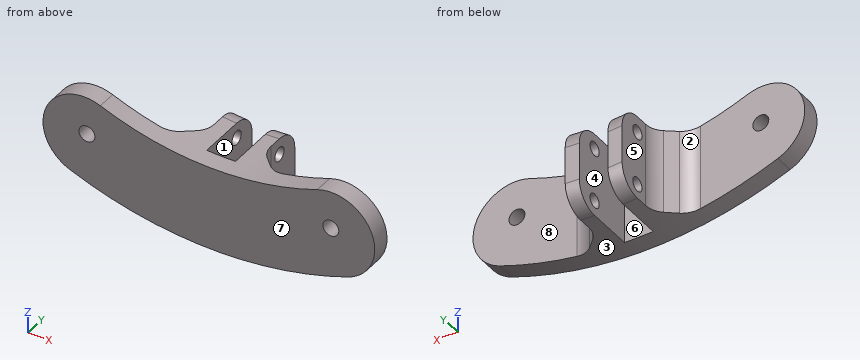
from build123d import *

# Parameters (mm, degrees)
SKETCH1_R               = 1.7
BOSS_EXTRUDE1_DEPTH     = 18.75
SKETCH2_W               = 29.270887873
SKETCH2_H               = 14.75
SKETCH2_W_2             = 6.11
CUT_EXTRUDE1_DEPTH      = 91.963568829
CHAMFER1_SIZE           = 5
FILLET1_R               = 5
CUT_EXTRUDE2_DEPTH      = 93.192977357
CUT_EXTRUDE2_DEPTH_BACK = 93.192977357
SKETCH4_R               = 1.5
FILLET2_R               = 5


with BuildPart() as part:
    # Sketch1 → Boss-Extrude1 (new body)
    with BuildSketch(Plane(origin=(0, 0, 0), x_dir=(1, 0, 0), z_dir=(0, 1, 0))):
        with BuildLine():
            ThreePointArc((-23.098921993, 59.418030115), (0, 63.75), (23.098921993, 59.418030115))
            ThreePointArc((23.098921993, 59.418030115), (34.716014466, 64.531190827), (29.602853754, 76.148283301))
            ThreePointArc((29.602853754, 76.148283301), (0, 81.7), (-29.602853754, 76.148283301))
            ThreePointArc((-29.602853754, 76.148283301), (-34.716014466, 64.531190827), (-23.098921993, 59.418030115))
        make_face()
        with Locations(Location((-25.965, 66.790526087, 0), (0, 0, 270))):
            Circle(SKETCH1_R, mode=Mode.SUBTRACT)
        with Locations(Location((25.965, 66.790526087, 0), (0, 0, 270))):
            Circle(SKETCH1_R, mode=Mode.SUBTRACT)
    extrude(amount=BOSS_EXTRUDE1_DEPTH)

    # Sketch2 → Cut-Extrude1 (cut, through all)
    with BuildSketch(Plane.XY):
        with Locations((-20.690443936, 11.375)):
            Rectangle(SKETCH2_W, SKETCH2_H)
        with Locations((20.690443936, 11.375)):
            Rectangle(SKETCH2_W, SKETCH2_H)
        with Locations((0, 11.375)):
            Rectangle(SKETCH2_W_2, SKETCH2_H)
    extrude(amount=-CUT_EXTRUDE1_DEPTH, mode=Mode.SUBTRACT)

    # Chamfer1
    chamfer1_edges = [part.edges().sort_by_distance(p)[0] for p in [
        (-6.055, 4, -72.468555262),
        (6.055, 4, -72.468555262),
    ]]
    chamfer(chamfer1_edges, length=CHAMFER1_SIZE)

    # Fillet1
    fillet1_edges = [part.edges().sort_by_distance(p)[0] for p in [
        (11.055, 4, -71.866378435),
        (6.055, 9, -72.468555262),
        (-11.055, 4, -71.866378435),
        (-6.055, 9, -72.468555262),
    ]]
    fillet(fillet1_edges, radius=FILLET1_R)

    # Sketch4 → Cut-Extrude2 (cut, two sides: drawn at the far end of the back side and taken through both)
    with BuildSketch(Plane.ZY.offset(-3.055).offset(-CUT_EXTRUDE2_DEPTH_BACK)):
        with Locations(Location((-78.409810047, 13.75, 0), (0, 0, 270))):
            Circle(SKETCH4_R)
        with Locations(Location((-66.909810047, 13.75, 0), (0, 0, 270))):
            Circle(SKETCH4_R)
    extrude(amount=CUT_EXTRUDE2_DEPTH + CUT_EXTRUDE2_DEPTH_BACK, mode=Mode.SUBTRACT)

    # Fillet2
    fillet2_edges = [part.edges().sort_by_distance(p)[0] for p in [
        (4.555770299, 18.75, -81.57288126),
        (-4.555770299, 18.75, -81.57288126),
        (-4.556267903, 18.75, -63.586971329),
        (4.556267903, 18.75, -63.586971329),
    ]]
    fillet(fillet2_edges, radius=FILLET2_R)


solid = part.part
Build history of the part. All positions in model axes, mm. Face numbers are marked on the shaded views. A direction names the side the tool comes from. Round coordinates to 2 decimals unless told otherwise and drop trailing zeros. Write each loop counter-clockwise with the first axis right and the second up, starting at its lowest first coordinate (ties: lowest second). Pieces come first, ordered by that corner, then holes. Notation, with made-up numbers: M 75.5,50 L 104.5,50 A24 ccw 104.5,88 Z; hole C -10,60.5 d10. An arc over 180 degrees is marked long. Use CSV: the item, a comma, the result in double quotes.
1. Two-plate mould, pull along X, no slides. Class the marked faces 1, 2, 3 and 4: +X half, -X half, draft (parallel to the pull), parting line (faces both ways), or undercut.
Reply:
face 1,"undercut"
face 2,"-X half"
face 3,"parting line"
face 4,"undercut"
2. Saw through at D-D (y = 8.75). Give the cut face in (x, z) (3 decimals), plus the area to 3 significant figures.
Reply:
outline,"M -6.626,-81.431 A81.7 ccw -3.055,-81.643 L -3.055,-63.677 A63.75 cw -6.626,-63.405 Z; M 3.055,-81.643 A81.7 ccw 6.626,-81.431 L 6.626,-63.405 A63.75 cw 3.055,-63.677 Z"
area,"129 mm²"
3. Flat gauge pins, fed straight in: pin 1 (6.5 mm diameter, centred on x = 1, z = -73.5, fed in from +Y); pin 2 (4 mm diameter, centred on x = -25.96, z = -66.79, fed in from +Y); pin 3 (4 mm diameter, centred on y = 13.5, z = -76.5, fed in from -X) (3 decimals); pin 4 (5 mm diameter, centred on y = 13.75, z = -78.41, fed in from +X) (3 decimals). Where does each tip first touch, or does it go through?
Reply:
pin 1,"stops at y = 18.75"
pin 2,"stops at y = 4"
pin 3,"stops at x = -6.055"
pin 4,"stops at x = 6.055"
4. Saw through at C-C (x = 12). Give the cut face in (y, z), plus the area to 3 significant figures.
Reply:
outline,"M 0,-80.81 L 4.13,-80.81 L 4.13,-62.61 L 0,-62.61 Z"
area,"75.2 mm²"
5. Saw through at A-A (y = 16.5). Give the cut face in (x, z) (3 decimals), plus the area to 3 significant figures.
Reply:
outline,"M -6.055,-80.649 A80.876 ccw -3.055,-80.818 L -3.055,-64.502 A64.574 cw -6.055,-64.29 Z; M 3.055,-80.818 A80.876 ccw 6.055,-80.649 L 6.055,-64.29 A64.574 cw 3.055,-64.502 Z"
area,"98.0 mm²"
6. Saw through at B-B (y = 3.25). Give the cut face in (x, z) (3 decimals), plus the area to 3 significant figures.
Reply:
outline,"M -29.603,-76.148 A81.7 ccw 29.603,-76.148 A8.975 ccw 23.099,-59.418 A63.75 cw -23.099,-59.418 A8.975 ccw Z; hole C -25.965,-66.791 d3.4; hole C 25.965,-66.791 d3.4"
area,"1,200 mm²"
7. Tool access for the marked faces 5, 6, 7 and 8: list every direction of +Z, -Z, +X, -X, +Y, -Y with a clear straight run to the whole face (end or side of a thin tool).
Reply:
face 5,"+Z, -Z, -X, +Y"
face 6,"+Z, -Z, +Y"
face 7,"+Z, -Z, +X, -X, -Y"
face 8,"+Z, -Z, +X, +Y"
8. Wall check: probe 1 along X at (y, z) = (15, -69.5) (3 decimals); probe 2 along Z at (x, y) = (-4.65, 13.75); probe 3 along X at (y, z) = (4.75, -80.5) (3 decimals). Give the ranges that are in metal, low to high. Write a range as from..to.
Reply:
probe 1,"x = -6.055..-3.055, 3.055..6.055"
probe 2,"z = -81.57..-79.91, -76.91..-68.41, -65.41..-63.58"
probe 3,"x = -10.492..-3.055, 3.055..10.492"
